```python
from build123d import *

# Parameters (mm, degrees)
ESQUISSE1_W             = 300
ESQUISSE1_H             = 180
BOSS_EXTRU_1_DEPTH      = 150
COQUE1_T                = -3
ENL_V_MAT_EXTRU_1_REACH = 5
ESQUISSE2_W             = 50
ESQUISSE2_H             = 122
ENL_V_MAT_EXTRU_2_REACH = 5
ESQUISSE3_W             = 30
ESQUISSE3_H             = 50


with BuildPart() as part:
    # Esquisse1 → Boss.-Extru.1 (new body)
    with BuildSketch(Plane.XY):
        with Locations((-150, 90)):
            Rectangle(ESQUISSE1_W, ESQUISSE1_H)
    extrude(amount=BOSS_EXTRU_1_DEPTH)

    # Coque1
    coque1_openings = [part.faces().sort_by_distance(p)[0] for p in [
        (-150, 90, 150),
    ]]
    offset(amount=COQUE1_T, openings=coque1_openings, kind=Kind.INTERSECTION)

    # Esquisse2 → Enlèv. mat.-Extru.1 (cut, up to next)
    with BuildSketch(Plane(origin=(0, 3, 0), x_dir=(1, 0, 0), z_dir=(0, 1, 0)), mode=Mode.PRIVATE) as enl_v_mat_extru_1_sk1:
        with Locations((-247, -64)):
            Rectangle(ESQUISSE2_W, ESQUISSE2_H)
    enl_v_mat_extru_1_tool1 = extrude(enl_v_mat_extru_1_sk1.sketch, amount=-ENL_V_MAT_EXTRU_1_REACH, mode=Mode.PRIVATE) & part.part
    add(enl_v_mat_extru_1_tool1.solids().sort_by_distance((-247, 3, 64))[0], mode=Mode.SUBTRACT)

    # Esquisse3 → Enlèv. mat.-Extru.2 (cut, up to next)
    with BuildSketch(Plane.XZ.offset(-177), mode=Mode.PRIVATE) as enl_v_mat_extru_2_sk1:
        with Locations((-78, 88)):
            Rectangle(ESQUISSE3_W, ESQUISSE3_H)
    enl_v_mat_extru_2_tool1 = extrude(enl_v_mat_extru_2_sk1.sketch, amount=-ENL_V_MAT_EXTRU_2_REACH, mode=Mode.PRIVATE) & part.part
    add(enl_v_mat_extru_2_tool1.solids().sort_by_distance((-78, 177, 88))[0], mode=Mode.SUBTRACT)


solid = part.part
```
CAD build for the part. Positions are in the model's coordinates, mm. A direction names the side the tool comes from. Round coordinates to 2 decimals unless told otherwise and drop trailing zeros. Order: outer loops, then holes, each group sorted by start corner. A loop starts at its lowest first (then second) coordinate and runs counter-clockwise, first axis right, second up. Notation, with made-up numbers: (7, -15) -> (16, -15) arc R20 cw to (16, 3) -> close; hole circle Ø5 at (25.5, 51). An arc over 180 degrees is marked (long way). One line per question, with ' | ' between items.
Q1. Drop flat-ended pins along their axis: pin 1 (1.5 mm diameter, centred on x = -162.5, z = 100.5, fed in from -Y); pin 2 (6 mm diameter, centred on x = -269, y = 79, fed in from +Z). Give the stop position or say it passes through.
Completed:
pin 1: stops at y = 0 | pin 2: stops at z = 3
Q2. Slice it at A-A (z = 79). Write the cut outline in (x, y), then the cut area to 3 significant figures.
Completed:
outline: (-300, 0) -> (-272, 0) -> (-272, 3) -> (-297, 3) -> (-297, 177) -> (-93, 177) -> (-93, 180) -> (-300, 180) -> close; (-222, 0) -> (0, 0) -> (0, 180) -> (-63, 180) -> (-63, 177) -> (-3, 177) -> (-3, 3) -> (-222, 3) -> close | area: 2,600 mm^2
Q3. Slice it at C-C (z = 136.5). Write the cut outline in (x, y), then the cut area to 3 significant figures.
Completed:
outline: (-300, 0) -> (0, 0) -> (0, 180) -> (-300, 180) -> close; hole (-297, 3) -> (-3, 3) -> (-3, 177) -> (-297, 177) -> close | area: 2,840 mm^2
Q4. Slice it at B-B (x = -265.5). Write the cut outline in (y, z).
Completed:
outline: (0, 0) -> (180, 0) -> (180, 150) -> (177, 150) -> (177, 3) -> (0, 3) -> close; (0, 125) -> (3, 125) -> (3, 150) -> (0, 150) -> close
Q5. Which spindle directions (+Z, -Z, +X, -X, +Y, -Y) get a long thin tool onto all of the face, cutting with end or side? Do faces 1 (the flat face through (-152, 91, 0)), 2 (the flat face through (-297, 89, 75)). Say none if no direction does.
Completed:
face 1: -Z, +X, -X, +Y, -Y | face 2: +Z
Q6. Two-plate mould, pull along Y, no slides. Class faces 3 (the flat face through (-300, 89, 74)), 4 (the flat face through (-3, 89, 75)), 5 (the flat face through (-152, 0, 74)): released by +Y, released by -Y, zero draft, split by the parting line, or undercut.
Completed:
face 3: zero draft | face 4: undercut | face 5: released by -Y
Q7. Slice it at D-D (y = 154.5). Write the cut outline in (x, z).
Completed:
outline: (-300, 0) -> (0, 0) -> (0, 150) -> (-3, 150) -> (-3, 3) -> (-297, 3) -> (-297, 150) -> (-300, 150) -> close
Q8. Probe probe 1 along X at (y, z) = (120, 49); probe 2 along Y at (x, z) = (-18, 46); probe 3 along Z at (x, y) = (-149.5, 62). List the from-to ranges inside material, lowest first.
Completed:
probe 1: x = -300 to -297, -3 to 0 | probe 2: y = 0 to 3, 177 to 180 | probe 3: z = 0 to 3
